Here's the drawing with two shaded views (mm, measured from the low corner). I have some questions. Give positions to 0.01 mm unless a question says otherwise; leave off trailing zeros. Write each loop counter-clockwise with the first axis right and the second up, starting at its lowest first coordinate (ties: lowest second). Pieces come first, ordered by that corner, then holes. Notation, with made-up numbers: (79, 48.25) -> (121, 48.25) arc R24 cw to (121, 60.25) -> close; hole circle Ø8 at (75.25, 27). An arc over 180 degrees is marked (long way). One line per item, written item: value.
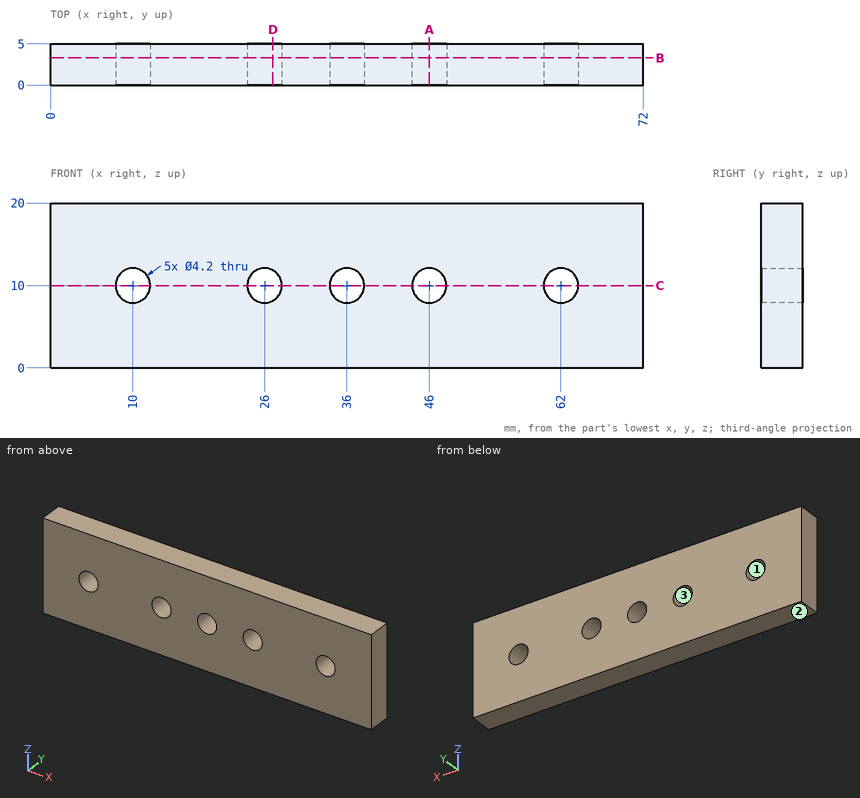
1) We'd pull the mould along X, two halves only. Please class the marked faces 1, 2 and 3: released by +X, released by -X, zero draft, split by the parting line, or undercut.
Answer list:
face 1: undercut
face 2: zero draft
face 3: undercut
2) If we section it at B-B (y = 3.3): Write out the boundary of the cut face in (x, z), and give its area (3 significant figures).
Answer list:
outline: (0, 0) -> (72, 0) -> (72, 20) -> (0, 20) -> close; hole circle Ø4.2 at (10, 10); hole circle Ø4.2 at (26, 10); hole circle Ø4.2 at (36, 10); hole circle Ø4.2 at (46, 10); hole circle Ø4.2 at (62, 10)
area: 1,370 mm^2
3) If we section it at C-C (z = 10): Write out the boundary of the cut face in (x, y).
Answer list:
outline: (0, 0) -> (7.9, 0) -> (7.9, 5) -> (0, 5) -> close; (12.1, 0) -> (23.9, 0) -> (23.9, 5) -> (12.1, 5) -> close; (28.1, 0) -> (33.9, 0) -> (33.9, 5) -> (28.1, 5) -> close; (38.1, 0) -> (43.9, 0) -> (43.9, 5) -> (38.1, 5) -> close; (48.1, 0) -> (59.9, 0) -> (59.9, 5) -> (48.1, 5) -> close; (64.1, 0) -> (72, 0) -> (72, 5) -> (64.1, 5) -> close
4) If we section it at D-D (x = 27): Write out the boundary of the cut face in (y, z), and give its area (3 significant figures).
Answer list:
outline: (0, 0) -> (5, 0) -> (5, 8.15) -> (0, 8.15) -> close; (0, 11.85) -> (5, 11.85) -> (5, 20) -> (0, 20) -> close
area: 81.5 mm^2
5) I need wall thicknesses on L1, parallel to X at y = 1.15, z = 10; L2, parallel to Z at x = 36, y = 1.5; L3, parallel to X at y = 4.35, z = 11.75. Which ranges of each line are inside material? Lowest first, please.
Answer list:
L1: x = 0 to 7.9, 12.1 to 23.9, 28.1 to 33.9, 38.1 to 43.9, 48.1 to 59.9, 64.1 to 72
L2: z = 0 to 7.9, 12.1 to 20
L3: x = 0 to 8.84, 11.16 to 24.84, 27.16 to 34.84, 37.16 to 44.84, 47.16 to 60.84, 63.16 to 72
6) If we section it at A-A (x = 46): Write out the boundary of the cut face in (y, z).
Answer list:
outline: (0, 0) -> (5, 0) -> (5, 7.9) -> (0, 7.9) -> close; (0, 12.1) -> (5, 12.1) -> (5, 20) -> (0, 20) -> close
